For this review, take the finished solid that the model builds, in its own axes (mm). Give positions to 0.01 mm unless a question says otherwise; leave off trailing zeros. Write each loop counter-clockwise with the first axis right and the second up, starting at its lowest first coordinate (ties: lowest second). Pieces come first, ordered by that corner, then holes. Notation, with made-up numbers: (-34, 14) -> (8, 14) arc R23 cw to (8, 26) -> close; hole circle Ø1 at (23, 17). An arc over 180 degrees is marked (long way). Write item = value, one per line.
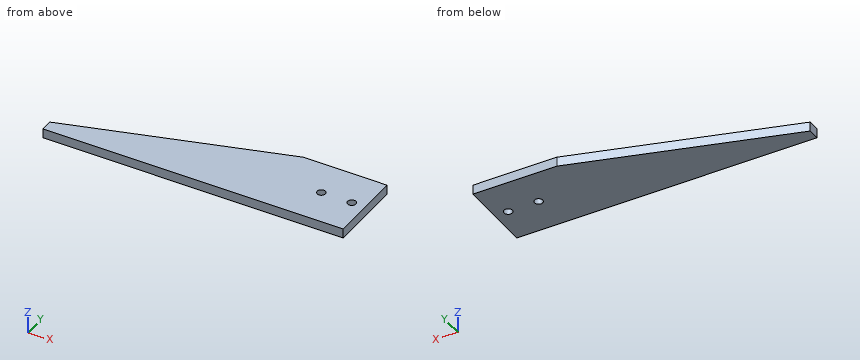
```python
from build123d import *

# Parameters (mm, degrees)
BOSS_EXTRUDE1_DEPTH = 6.35
SKETCH2_R           = 2.778125
CUT_EXTRUDE1_DEPTH  = 208.258653961


with BuildPart() as part:
    # Sketch1 → Boss-Extrude1 (new body)
    with BuildSketch(Plane.XY):
        Polygon((0, 0), (0, 50.8), (-56.115509559, 50.8), (-200.836219696, 7.8694881), (-200.836219696, 0), align=None)
    extrude(amount=BOSS_EXTRUDE1_DEPTH)

    # Sketch2 → Cut-Extrude1 (cut, through all)
    with BuildSketch(Plane.XY.offset(6.35)):
        with Locations((-29.21, 25.4)):
            Circle(SKETCH2_R)
        with Locations((-8.89, 25.4)):
            Circle(SKETCH2_R)
    extrude(amount=-CUT_EXTRUDE1_DEPTH, mode=Mode.SUBTRACT)


solid = part.part
```
(1) Take a section at A-A (x = -8.89). Write out the cut boundary in (y, z).
Answers below:
outline = (0, 0) -> (22.62, 0) -> (22.62, 6.35) -> (0, 6.35) -> close; (28.18, 0) -> (50.8, 0) -> (50.8, 6.35) -> (28.18, 6.35) -> close
(2) To check wall thickness, follow probe 1 along Y at (x, z) = (-8.89, 4.75); probe 2 along Y at (x, z) = (-151, 2); probe 3 along Y at (x, z) = (-114, 1.25). State the ranges of each line that lie inside material, in increasing order.
Answers below:
probe_1 = 0 to 22.62, 28.18 to 50.8
probe_2 = 0 to 22.65
probe_3 = 0 to 33.63
(3) Take a section at C-C (y = 25.4). Write out the cut boundary in (x, z).
Answers below:
outline = (-141.74, 0) -> (-31.99, 0) -> (-31.99, 6.35) -> (-141.74, 6.35) -> close; (-26.43, 0) -> (-11.67, 0) -> (-11.67, 6.35) -> (-26.43, 6.35) -> close; (-6.11, 0) -> (0, 0) -> (0, 6.35) -> (-6.11, 6.35) -> close
(4) Take a section at D-D (y = 41.5). Write out the cut boundary in (x, z), plus the area to 3 significant figures.
Answers below:
outline = (-87.47, 0) -> (0, 0) -> (0, 6.35) -> (-87.47, 6.35) -> close
area = 555 mm^2
(5) Take a section at B-B (z = 2.25). Write out the cut boundary in (x, y), plus the area to 3 significant figures.
Answers below:
outline = (-200.84, 0) -> (0, 0) -> (0, 50.8) -> (-56.12, 50.8) -> (-200.84, 7.87) -> close; hole circle Ø5.56 at (-29.21, 25.4); hole circle Ø5.56 at (-8.89, 25.4)
area = 7,050 mm^2
(6) For pin 1 (4.5 mm diameter, centred on x = -29.21, y = 25.4, fed in from +Z); pin 2 (2 mm diameter, centred on x = -158, z = 1.5, fed in from +Y), all flat-tipped, find the tip position at first contact; note any pin that passes through.
Answers below:
pin_1 = through
pin_2 = 20.87
